CAD build for the part. Positions are in the model's coordinates, mm. Coordinates: 2 decimals unless noted, no trailing zeros. Order: outer loops, then holes, each group sorted by start corner. A loop starts at its lowest first (then second) coordinate and runs counter-clockwise, first axis right, second up. Notation, with made-up numbers: M 26.25,-21.75 L 38.25,-21.75 A18 ccw 38.25,2.25 Z; hole C -36.5,-33 d1. An arc over 180 degrees is marked long. One line per item, written item: value.
from build123d import *

# Parameters (mm, degrees)
SKETCH1_W           = 295
SKETCH1_H           = 125
BOSS_EXTRUDE1_DEPTH = 2.5
FILLET1_R           = 7.5
FILLET2_R           = 1
CUT_EXTRUDE4_DEPTH  = 10


with BuildPart() as part:
    # Sketch1 → Boss-Extrude1 (new body)
    with BuildSketch(Plane(origin=(0, 0, 0), x_dir=(1, 0, 0), z_dir=(0, 1, 0))):
        Rectangle(SKETCH1_W, SKETCH1_H)
    extrude(amount=BOSS_EXTRUDE1_DEPTH)

    # Fillet1
    fillet1_edges = [part.edges().sort_by_distance(p)[0] for p in [
        (147.5, 1.25, 62.5),
        (-147.5, 1.25, 62.5),
        (-147.5, 1.25, -62.5),
        (147.5, 1.25, -62.5),
    ]]
    fillet(fillet1_edges, radius=FILLET1_R)

    # Fillet2
    fillet2_edges = [part.edges().sort_by_distance(p)[0] for p in [
        (147.5, 2.5, 0),
        (0, 2.5, 62.5),
        (0, 2.5, -62.5),
        (-147.5, 2.5, 0),
        (-145.303300859, 2.5, -60.303300859),
        (145.303300859, 2.5, -60.303300859),
        (-145.303300859, 2.5, 60.303300859),
        (145.303300859, 2.5, 60.303300859),
    ]]
    fillet(fillet2_edges, radius=FILLET2_R)

    # Sketch4 → Cut-Extrude4 (cut)
    with BuildSketch(Plane(origin=(0, 2.5, 0), x_dir=(1, 0, 0), z_dir=(0, 1, 0))):
        with BuildLine():
            Line((-33.073998348, 3.090010623), (-75.025380216, 0.395089537))
            ThreePointArc((-75.025380216, 0.395089537), (-75.3959039, 0), (-75.025380216, -0.395089537))
            Line((-75.025380216, -0.395089537), (-33.073998348, -3.090010623))
            ThreePointArc((-33.073998348, -3.090010623), (-16.332033074, -8.52386445), (-4.236704547, -21.311483324))
            ThreePointArc((-4.236704547, -21.311483324), (0, -23.802100242), (4.236704547, -21.311483324))
            ThreePointArc((4.236704547, -21.311483324), (16.332033074, -8.52386445), (33.073998348, -3.090010623))
            Line((33.073998348, -3.090010623), (75.025380216, -0.395089537))
            ThreePointArc((75.025380216, -0.395089537), (75.3959039, 0), (75.025380216, 0.395089537))
            Line((75.025380216, 0.395089537), (33.073998348, 3.090010623))
            ThreePointArc((33.073998348, 3.090010623), (16.332033074, 8.52386445), (4.236704547, 21.311483324))
            ThreePointArc((4.236704547, 21.311483324), (0, 23.802100242), (-4.236704547, 21.311483324))
            ThreePointArc((-4.236704547, 21.311483324), (-16.332033074, 8.52386445), (-33.073998348, 3.090010623))
        make_face()
    extrude(amount=-CUT_EXTRUDE4_DEPTH, mode=Mode.SUBTRACT)


solid = part.part
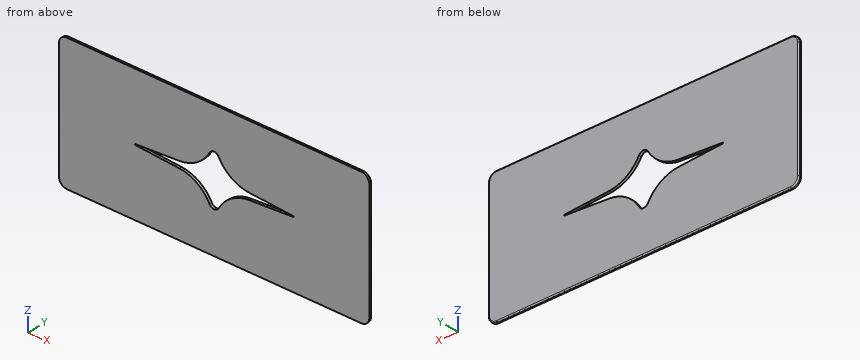
Q1. Slice it at C-C (z = -13). List the corners of the cut face in (x, y), plus the area to 3 significant figures.
Recorded:
outline: M -147.5,0 L -10.63,0 L -10.63,2.5 L -146.5,2.5 A1 ccw -147.5,1.5 Z; M 10.63,0 L 147.5,0 L 147.5,1.5 A1 ccw 146.5,2.5 L 10.63,2.5 Z
area: 684 mm^2
Q2. Slice it at B-B (x = 53). List the corners of the cut face in (y, z).
Recorded:
outline: M 0,-62.5 L 1.5,-62.5 A1 ccw 2.5,-61.5 L 2.5,-1.81 L 0,-1.81 Z; M 0,1.81 L 2.5,1.81 L 2.5,61.5 A1 ccw 1.5,62.5 L 0,62.5 Z
Q3. Slice it at A-A (y = 1.1). List the corners of the cut face in (x, z).
Recorded:
outline: M -147.5,-55 A7.5 ccw -140,-62.5 L 140,-62.5 A7.5 ccw 147.5,-55 L 147.5,55 A7.5 ccw 140,62.5 L -140,62.5 A7.5 ccw -147.5,55 Z; hole M -75.03,-0.4 L -33.07,-3.09 A35.62 cw -4.24,-21.31 A4.85 ccw 4.24,-21.31 A35.62 cw 33.07,-3.09 L 75.03,-0.4 A0.4 ccw 75.03,0.4 L 33.07,3.09 A35.62 cw 4.24,21.31 A4.85 ccw -4.24,21.31 A35.62 cw -33.07,3.09 L -75.03,0.4 A0.4 ccw Z
Q4. Drill centre lines: line 1 along X through (y, z) = (0.15, 11.5); line 2 along Z through (x, y) = (21, 0.5); line 3 along Z through (x, y) = (-37.5, 2.3). Where is each one in solid material? Low to high.
Recorded:
line 1: x = -147.5 to -12.29, 12.29 to 147.5
line 2: z = -62.5 to -6.04, 6.04 to 62.5
line 3: z = -62.1 to -2.81, 2.81 to 62.1
